The listing builds one solid part. Answer for the finished solid, in the listing's coordinates (mm). Coordinates: 2 decimals unless noted, no trailing zeros. Order: outer loops, then holes, each group sorted by start corner. A loop starts at its lowest first (then second) coordinate and runs counter-clockwise, first axis right, second up. Notation, with made-up numbers: (53.5, 38.5) -> (106.5, 38.5) arc R13 cw to (106.5, 42.5) -> close; hole circle Ø1 at (71.25, 29). An arc over 180 degrees is marked (long way). One line per question, with ' | ' between items.
from build123d import *

# Parameters (mm, degrees)
SKETCH_W        = 286
SKETCH_H        = 250
PAD_DEPTH       = 6
SKETCH001_R     = 1.7
SKETCH001_W     = 22
SKETCH001_H     = 6
SKETCH001_W_2   = 26
SKETCH001_H_2   = 35
POCKET_DEPTH    = 765.822032
SKETCH002_R     = 1.7
SKETCH002_W     = 6
SKETCH002_H     = 10
POCKET001_DEPTH = 765.822032
SKETCH003_R     = 1.7
POCKET002_DEPTH = 6.001
SKETCH004_R     = 13.25
SKETCH004_R_2   = 1.7
POCKET003_DEPTH = 765.822032
SKETCH005_R     = 1.7
POCKET004_DEPTH = 6.001
POCKET005_DEPTH = 765.822032
SKETCH007_R     = 1.21
HOLE_DEPTH      = 765.822032
POCKET006_DEPTH = 765.822032
SKETCH009_R     = 4
SKETCH009_R_2   = 1.6
POCKET007_DEPTH = 6.001


with BuildPart() as part:
    # Sketch → Pad (new body)
    with BuildSketch(Plane.XY):
        Rectangle(SKETCH_W, SKETCH_H)
    extrude(amount=PAD_DEPTH)

    # Sketch001 (on Face6 of Pad) → Pocket (cut, through all)
    with BuildSketch(Plane.XY.offset(6)):
        with Locations((-38, 27)):
            Circle(SKETCH001_R)
        with Locations((0, 27)):
            Circle(SKETCH001_R)
        with Locations((38, 27)):
            Circle(SKETCH001_R)
        with Locations((-22, 27)):
            Rectangle(SKETCH001_W, SKETCH001_H)
        with Locations((22, 27)):
            Rectangle(SKETCH001_W, SKETCH001_H)
        with Locations((-62, 17.5)):
            Rectangle(SKETCH001_W_2, SKETCH001_H_2)
        with Locations((62, 17.5)):
            Rectangle(SKETCH001_W_2, SKETCH001_H_2)
    pocket = extrude(amount=-POCKET_DEPTH, mode=Mode.SUBTRACT)

    # Mirrored: Pocket across Sketch001 H_Axis
    add(pocket.mirror(Plane(origin=(0, 0, 6), x_dir=(0, 0, 1), z_dir=(0, 1, 0))), mode=Mode.SUBTRACT)

    # Sketch002 (on Face5 of Mirrored) → Pocket001 (cut, through all)
    with BuildSketch(Plane.XY.offset(6)):
        with Locations((-125, 49.7)):
            Circle(SKETCH002_R)
        with Locations((-109, 49.7)):
            Circle(SKETCH002_R)
        Polygon((-136, 26), (-136, -26), (-75, -26), (-75, 26), (-112, 26), (-112, 29.7), (-106, 29.7), (-106, 39.7), (-112, 39.7), (-112, 56), (-122, 56), (-122, 39.7), (-128, 39.7), (-128, 29.7), (-122, 29.7), (-122, 26), align=None)
        with Locations((-125, 64.7)):
            Rectangle(SKETCH002_W, SKETCH002_H)
        with Locations((-109, 64.7)):
            Rectangle(SKETCH002_W, SKETCH002_H)
    pocket001 = extrude(amount=-POCKET001_DEPTH, mode=Mode.SUBTRACT)

    # Mirrored001: Pocket001 across Sketch002 V_Axis
    add(pocket001.mirror(Plane(origin=(0, 0, 6), x_dir=(0, 0, 1), z_dir=(1, 0, 0))), mode=Mode.SUBTRACT)

    # Sketch003 (on Face5 of Mirrored001) → Pocket002 (cut, through all)
    with BuildSketch(Plane.XY.offset(6)):
        with Locations((-40, 65)):
            Circle(SKETCH003_R)
        with Locations((40, 65)):
            Circle(SKETCH003_R)
    extrude(amount=-POCKET002_DEPTH, mode=Mode.SUBTRACT)

    # Sketch004 → Pocket003 (cut, through all)
    with BuildSketch(Plane.XY.offset(6)):
        with Locations((0, 108)):
            Circle(SKETCH004_R)
        with Locations((0, 88.25)):
            Circle(SKETCH004_R_2)
        with Locations((0, 55.65)):
            Circle(SKETCH004_R_2)
        with Locations((0, 65.65)):
            Circle(SKETCH004_R_2)
    pocket003 = extrude(amount=-POCKET003_DEPTH, mode=Mode.SUBTRACT)

    # Sketch005 → Pocket004 (cut, through all)
    with BuildSketch(Plane.XY.offset(6)):
        with Locations((135, 80)):
            Circle(SKETCH005_R)
        with Locations((-135, 80)):
            Circle(SKETCH005_R)
        with Locations((-135, -80)):
            Circle(SKETCH005_R)
        with Locations((135, -80)):
            Circle(SKETCH005_R)
    extrude(amount=-POCKET004_DEPTH, mode=Mode.SUBTRACT)

    # Sketch006 (on Face5 of Pocket004) → Pocket005 (cut, through all)
    with BuildSketch(Plane.XY.offset(6)):
        with BuildLine():
            Line((-143, -115), (-143, -125))
            Line((-143, -125), (-133, -125))
            ThreePointArc((-143, -115), (-140.071068, -122.071068), (-133, -125))
        make_face()
        with BuildLine():
            Line((143, -115), (143, -125))
            Line((143, -125), (133, -125))
            ThreePointArc((133, -125), (140.071068, -122.071068), (143, -115))
        make_face()
    pocket005 = extrude(amount=-POCKET005_DEPTH, mode=Mode.SUBTRACT)

    # Mirrored004: Pocket005 across Sketch006 H_Axis
    add(pocket005.mirror(Plane(origin=(0, 0, 6), x_dir=(0, 0, 1), z_dir=(0, 1, 0))), mode=Mode.SUBTRACT)

    # Sketch007 (on Face4 of Mirrored004) → Hole (cut, through all)
    with BuildSketch(Plane.XY.offset(6)):
        with Locations((-127.5, -116.2)):
            Circle(SKETCH007_R)
        with Locations((-118, -116.2)):
            Circle(SKETCH007_R)
        with Locations((127.5, -116.2)):
            Circle(SKETCH007_R)
        with Locations((118, -116.2)):
            Circle(SKETCH007_R)
    hole = extrude(amount=-HOLE_DEPTH, mode=Mode.SUBTRACT)

    # Mirrored005: Hole across Sketch007 H_Axis
    add(hole.mirror(Plane(origin=(0, 0, 6), x_dir=(0, 0, 1), z_dir=(0, 1, 0))), mode=Mode.SUBTRACT)

    # Sketch008 (on Face4 of Mirrored005) → Pocket006 (cut, through all)
    with BuildSketch(Plane.XY.offset(6)):
        Polygon((-4, -143.30127), (-79, -100), (-154, -143.30127), (-154, -229.903811), (-79, -273.205081), (-4, -229.903811), align=None)
        Polygon((4, -143.30127), (4, -229.903811), (79, -273.205081), (154, -229.903811), (154, -143.30127), (79, -100), align=None)
    pocket006 = extrude(amount=-POCKET006_DEPTH, mode=Mode.SUBTRACT)

    # Mirrored006: Pocket006 across Sketch008 H_Axis
    add(pocket006.mirror(Plane(origin=(0, 0, 6), x_dir=(0, 0, 1), z_dir=(0, 1, 0))), mode=Mode.SUBTRACT)

    # Sketch009 (on Face4 of Mirrored006) → Pocket007 (cut, through all)
    with BuildSketch(Plane.XY.offset(6)):
        with Locations((0, -63.85)):
            Circle(SKETCH009_R)
        with Locations((-18.5, -63.85)):
            Circle(SKETCH009_R_2)
        with Locations((18.5, -63.85)):
            Circle(SKETCH009_R_2)
    extrude(amount=-POCKET007_DEPTH, mode=Mode.SUBTRACT)

    # Mirrored007: Pocket003 across Sketch004 H_Axis
    add(pocket003.mirror(Plane(origin=(0, 0, 6), x_dir=(0, 0, 1), z_dir=(0, 1, 0))), mode=Mode.SUBTRACT)


solid = part.part
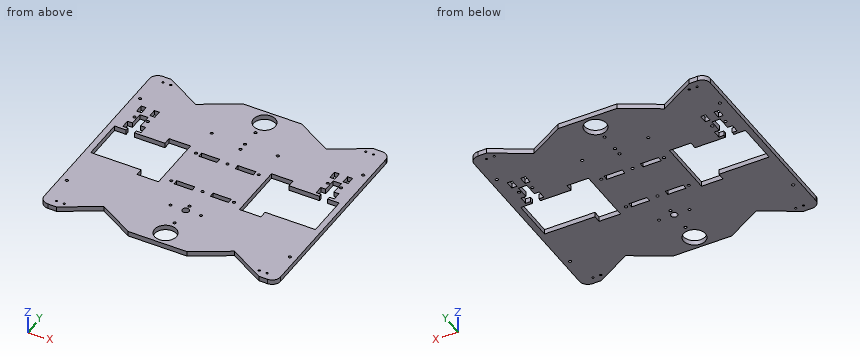
Item 1: Section B-B, the plane y = -4 is taken. Give the vertices of the cut face in (x, z), plus the area to 3 significant figures.
Computed values:
outline: (-143, 0) -> (-136, 0) -> (-136, 6) -> (-143, 6) -> close; (-49, 0) -> (49, 0) -> (49, 6) -> (-49, 6) -> close; (136, 0) -> (143, 0) -> (143, 6) -> (136, 6) -> close | area: 672 mm^2
Item 2: Find the intervals of material crossed by L1, parallel to X at y = 5.5, z = 5.35; L2, parallel to X at y = -79, z = 1.25; L3, parallel to Y at x = -135, z = 3.3, in increasing order.
Computed values:
L1: x = -143 to -136, -49 to 49, 136 to 143 | L2: x = -143 to -136.37, -133.63 to 133.63, 136.37 to 143 | L3: y = -124.8 to -81.7, -78.3 to -26, 26 to 78.3, 81.7 to 124.8
Item 3: Section C-C, the plane x = 67 is taken. Give the vertices of the cut face in (y, z), plus the area to 3 significant figures.
Computed values:
outline: (-106.93, 0) -> (-35, 0) -> (-35, 6) -> (-106.93, 6) -> close; (35, 0) -> (106.93, 0) -> (106.93, 6) -> (35, 6) -> close | area: 863 mm^2
Item 4: Section A-A, the plane x = 25 is taken. Give the vertices of the cut face in (y, z).
Computed values:
outline: (-125, 0) -> (-30, 0) -> (-30, 6) -> (-125, 6) -> close; (-24, 0) -> (24, 0) -> (24, 6) -> (-24, 6) -> close; (30, 0) -> (125, 0) -> (125, 6) -> (30, 6) -> close
Item 5: Section D-D, the plane y = 108 is taken. Give the vertices of the cut face in (x, z).
Computed values:
outline: (-143, 0) -> (-92.86, 0) -> (-92.86, 6) -> (-143, 6) -> close; (-65.14, 0) -> (-13.25, 0) -> (-13.25, 6) -> (-65.14, 6) -> close; (13.25, 0) -> (65.14, 0) -> (65.14, 6) -> (13.25, 6) -> close; (92.86, 0) -> (143, 0) -> (143, 6) -> (92.86, 6) -> close
Item 6: Each of these flat-tipped pins is pushed along its axis until it touches: pin 1 Ø1.9 at (x, y) = (-118, -116.2) entering from +Z; pin 2 Ø1.8 at (x, z) = (-108.5, 2.5) entering from +Y; pin 3 Ø3.5 at (x, y) = (-18.5, -63.85) entering from +Z. Where does it stop, or does it pass through?
Computed values:
pin 1: passes through | pin 2: stops at y = 117.55 | pin 3: stops at z = 6
